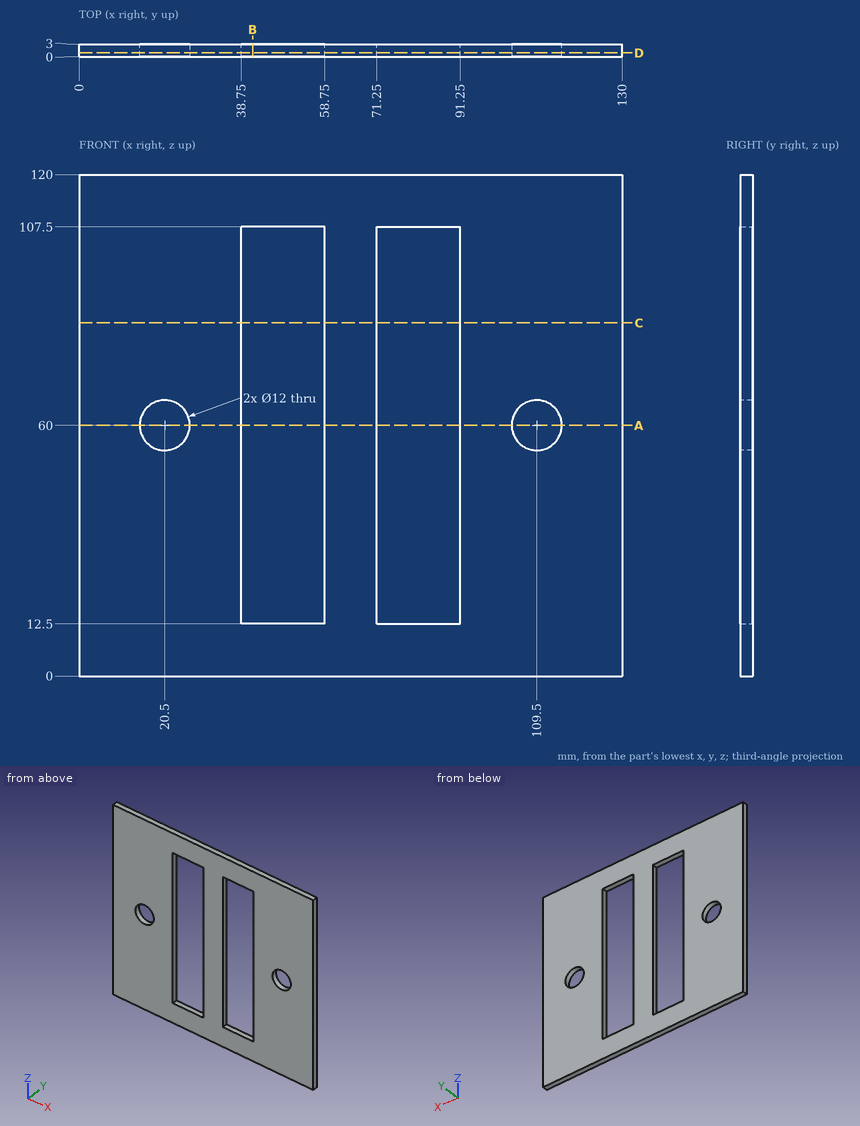
Print and shaded views of the part. All mm, measured from the part's lowest x, y and z. Coordinates: 2 decimals unless noted, no trailing zeros. Write each loop counter-clockwise with the first axis right and the second up, starting at its lowest first coordinate (ties: lowest second). Pieces come first, ordered by that corner, then holes. Notation, with made-up numbers: (-19, 67.5) -> (2, 67.5) arc R24 ccw to (2, 83.5) -> close; hole circle Ø4 at (73, -26). An arc over 180 degrees is marked (long way). Use CSV: the item, a comma, the result in double quotes. Start each with the question number.
Q1. Drill centre lines: probe 1 along X at (y, z) = (1.2, 82); probe 2 along Z at (x, y) = (109.5, 1.25); probe 3 along X at (y, z) = (0.4, 56). Where is each one in solid material? Low to high.
Q2. Cut at C-C, the plane z = 84.5. List the corners of the cut face in (x, y), then the cut area to 3 significant figures.
Q3. Cut at B-B, the plane x = 41.5. List the corners of the cut face in (y, z), then the cut area to 3 significant figures.
Q4. Cut at A-A, the plane z = 60. List the corners of the cut face in (x, y), then the cut area to 3 significant figures.
Q5. Cut at D-D, the plane y = 0.9. List the corners of the cut face in (x, z).
Checked values:
1,probe 1,"x = 0 to 38.75, 58.75 to 71.25, 91.25 to 130"
1,probe 2,"z = 0 to 54, 66 to 120"
1,probe 3,"x = 0 to 16.03, 24.97 to 38.75, 58.75 to 71.25, 91.25 to 105.03, 113.97 to 130"
2,outline,"(0, 0) -> (38.75, 0) -> (38.75, 3) -> (0, 3) -> close; (58.75, 0) -> (71.25, 0) -> (71.25, 3) -> (58.75, 3) -> close; (91.25, 0) -> (130, 0) -> (130, 3) -> (91.25, 3) -> close"
2,area,"270 mm²"
3,outline,"(0, 0) -> (3, 0) -> (3, 12.5) -> (0, 12.5) -> close; (0, 107.5) -> (3, 107.5) -> (3, 120) -> (0, 120) -> close"
3,area,"75.0 mm²"
4,outline,"(0, 0) -> (14.5, 0) -> (14.5, 3) -> (0, 3) -> close; (26.5, 0) -> (38.75, 0) -> (38.75, 3) -> (26.5, 3) -> close; (58.75, 0) -> (71.25, 0) -> (71.25, 3) -> (58.75, 3) -> close; (91.25, 0) -> (103.5, 0) -> (103.5, 3) -> (91.25, 3) -> close; (115.5, 0) -> (130, 0) -> (130, 3) -> (115.5, 3) -> close"
4,area,"198 mm²"
5,outline,"(0, 0) -> (130, 0) -> (130, 120) -> (0, 120) -> close; hole circle Ø12 at (20.5, 60); hole (38.75, 12.5) -> (58.75, 12.5) -> (58.75, 107.5) -> (38.75, 107.5) -> close; hole (71.25, 12.5) -> (91.25, 12.5) -> (91.25, 107.5) -> (71.25, 107.5) -> close; hole circle Ø12 at (109.5, 60)"
